Check sheet for the modelled part. Datum: model origin and axes. Units: mm. Coordinates: 2 decimals unless noted, no trailing zeros. Write each loop counter-clockwise with the first axis right and the second up, starting at its lowest first coordinate (ties: lowest second). Pieces come first, ordered by that corner, then holes. Notation, with made-up numbers: M -22,17.5 L -6,17.5 A19 cw -6,21.5 Z; hole C 46.5,51 d5. An arc over 180 degrees is marked long. Answer as CSV lines item,"result". Start each with the question number.
Q1. Depth check by flat-ended pin: pin 1 Ø3 at (x, y) = (-119.5, -28) entering from -Z. Enter the tip coordinate at first touch or a pass-through.
Q2. Sectioned sample at A-A, the plane y = -17.5. Record the cut outline in (x, z), then the cut area to 3 significant figures.
Q3. Thickness scan on line 1 along Y through (x, z) = (-47.5, 16.5); line 2 along X through (y, z) = (-10, 15); line 3 along Y through (x, z) = (-184.5, 19.75). Record the ranges inside material, lowest first. Write a range as from..to.
from build123d import *

# Parameters (mm, degrees)
F0_W     = 600
F0_H     = 157
F1_DEPTH = 25
F3_DEPTH = 12
F5_DEPTH = 545
F6_DEPTH = 16


with BuildPart() as f1:
    # F0 (on Top) → F1 (new body)
    with BuildSketch(Plane.XY):
        with Locations((0, 23.160652)):
            Rectangle(F0_W, F0_H)
    extrude(amount=F1_DEPTH)

    # F2 (on face) → F3 (cut)
    with BuildSketch(Plane.XY.offset(25)):
        with BuildLine():
            Line((-270, 91.660652), (-285, 91.660652))
            ThreePointArc((-285, 91.660652), (-288.535534, 90.196186), (-290, 86.660652))
            Line((-290, 86.660652), (-290, -40.339348))
            ThreePointArc((-290, -40.339348), (-288.535534, -43.874882), (-285, -45.339348))
            Line((-285, -45.339348), (-270, -45.339348))
            ThreePointArc((-270, -45.339348), (-266.464466, -43.874882), (-265, -40.339348))
            Line((-265, -40.339348), (-265, 86.660652))
            ThreePointArc((-265, 86.660652), (-266.464466, 90.196186), (-270, 91.660652))
        make_face()
        with BuildLine():
            ThreePointArc((285, -45.339348), (288.535534, -43.874882), (290, -40.339348))
            Line((290, -40.339348), (290, 86.660652))
            ThreePointArc((290, 86.660652), (288.535534, 90.196186), (285, 91.660652))
            Line((285, 91.660652), (270, 91.660652))
            ThreePointArc((270, 91.660652), (266.464466, 90.196186), (265, 86.660652))
            Line((265, 86.660652), (265, -40.339348))
            ThreePointArc((265, -40.339348), (266.464466, -43.874882), (270, -45.339348))
            Line((270, -45.339348), (285, -45.339348))
        make_face()
    extrude(amount=-F3_DEPTH, mode=Mode.SUBTRACT)

    # F4 (on face) → F5 (cut)
    with BuildSketch(Plane.YZ.offset(265)):
        Polygon((-30.339348, 25), (-40.339348, 25), (-40.339348, 18.5), (-44.339348, 18.5), (-44.339348, 13), (-26.339348, 13), (-26.339348, 18.5), (-30.339348, 18.5), align=None)
        Polygon((-1.339348, 25), (-1.339348, 18.5), (-5.339348, 18.5), (-5.339348, 13), (12.660652, 13), (12.660652, 18.5), (8.660652, 18.5), (8.660652, 25), align=None)
        Polygon((37.660652, 25), (37.660652, 18.5), (33.660652, 18.5), (33.660652, 13), (51.660652, 13), (51.660652, 18.5), (47.660652, 18.5), (47.660652, 25), align=None)
        Polygon((76.660652, 25), (76.660652, 18.5), (72.660652, 18.5), (72.660652, 13), (90.660652, 13), (90.660652, 18.5), (86.660652, 18.5), (86.660652, 25), align=None)
    extrude(amount=-F5_DEPTH, mode=Mode.SUBTRACT)

    # F4 (on face) → F6 (cut)
    with BuildSketch(Plane.YZ.offset(265)):
        Polygon((-30.339348, 25), (-40.339348, 25), (-40.339348, 18.5), (-44.339348, 18.5), (-44.339348, 13), (-26.339348, 13), (-26.339348, 18.5), (-30.339348, 18.5), align=None)
        Polygon((-1.339348, 25), (-1.339348, 18.5), (-5.339348, 18.5), (-5.339348, 13), (12.660652, 13), (12.660652, 18.5), (8.660652, 18.5), (8.660652, 25), align=None)
        Polygon((37.660652, 25), (37.660652, 18.5), (33.660652, 18.5), (33.660652, 13), (51.660652, 13), (51.660652, 18.5), (47.660652, 18.5), (47.660652, 25), align=None)
        Polygon((76.660652, 25), (76.660652, 18.5), (72.660652, 18.5), (72.660652, 13), (90.660652, 13), (90.660652, 18.5), (86.660652, 18.5), (86.660652, 25), align=None)
    extrude(amount=F6_DEPTH, mode=Mode.SUBTRACT)


solid = f1.part
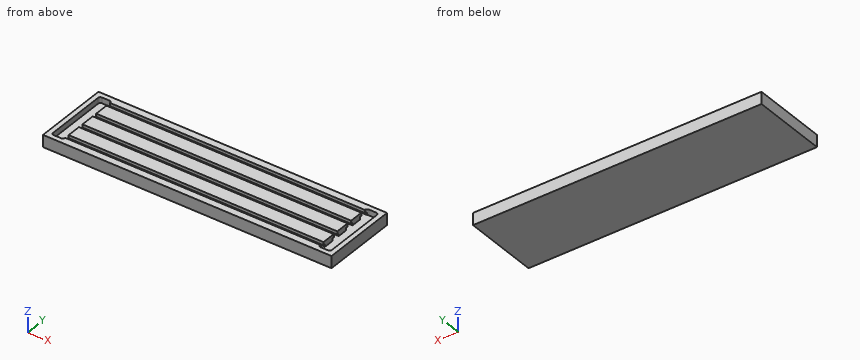
Output:
1,pin 1,"stops at z = 0"
2,outline,"M -300,0 L 300,0 L 300,25 L 290,25 L 290,13 L 265,13 L 265,25 L -265,25 L -265,13 L -290,13 L -290,25 L -300,25 Z"
2,area,"14,400 mm^2"
3,line 1,"y = -55.34..-44.34, -26.34..-5.34, 12.66..33.66, 51.66..72.66, 90.66..101.66"
3,line 2,"x = -300..-290, -265..265, 290..300"
3,line 3,"y = -55.34..-40.34, -30.34..-1.34, 8.66..37.66, 47.66..76.66, 86.66..101.66"
